from build123d import *

# Parameters (mm, degrees)
EXTRUDE_1_DEPTH     = 50
CHAMFER_1_SIZE      = 5
FILLET_1_R          = 1
SKETCH_2_R          = 12.5
SKETCH_2_R_2        = 2.147801841
CUT_EXTRUDE_1_DEPTH = 84.432542833
CUT_EXTRUDE_2_DEPTH = 80.287617379


with BuildPart() as part:
    # 스케치1 → 보스-돌출1 (new body)
    with BuildSketch(Plane(origin=(0, 0, 0), x_dir=(0, 0, -1), z_dir=(1, 0, 0))):
        with BuildLine():
            Line((-18.568527919, -10.355329949), (31.431472081, -10.355329949))
            ThreePointArc((31.431472081, -10.355329949), (33.552792425, -9.476650293), (34.431472081, -7.355329949))
            Line((34.431472081, -7.355329949), (34.431472081, 40.644670051))
            Line((34.431472081, 40.644670051), (31.431472081, 40.644670051))
            Line((31.431472081, 40.644670051), (31.431472081, -7.355329949))
            Line((31.431472081, -7.355329949), (-18.568527919, -7.355329949))
            Line((-18.568527919, -7.355329949), (-18.568527919, -10.355329949))
        make_face()
    extrude(amount=EXTRUDE_1_DEPTH)

    # 모따기1
    chamfer_1_edges = [part.edges().sort_by_distance(p)[0] for p in [
        (0, -8.855329949, 18.568527919),
        (50, 40.644670051, -32.931472081),
        (50, -8.855329949, 18.568527919),
        (0, 40.644670051, -32.931472081),
    ]]
    chamfer(chamfer_1_edges, length=CHAMFER_1_SIZE)

    # 필렛1
    fillet_1_edges = [part.edges().sort_by_distance(p)[0] for p in [
        (25, -7.355329949, -31.431472081),
    ]]
    fillet(fillet_1_edges, radius=FILLET_1_R)

    # 스케치2 → 컷-돌출1 (cut, through all)
    with BuildSketch(Plane(origin=(0, 0, -34.431472081), x_dir=(-1, 0, 0), z_dir=(0, 0, -1))):
        with Locations((-25, 19.644670051)):
            Circle(SKETCH_2_R)
        with Locations((-37.374368671, 32.019038722)):
            Circle(SKETCH_2_R_2)
        with Locations(Location((-12.625631329, 32.019038722, 0), (0, 0, 90))):
            Circle(SKETCH_2_R_2)
        with Locations((-12.625631329, 7.27030138)):
            Circle(SKETCH_2_R_2)
        with Locations(Location((-37.374368671, 7.27030138, 0), (0, 0, 90))):
            Circle(SKETCH_2_R_2)
    extrude(amount=-CUT_EXTRUDE_1_DEPTH, mode=Mode.SUBTRACT)

    # 스케치3 → 컷-돌출2 (cut, through all)
    with BuildSketch(Plane.XZ.offset(10.355329949)):
        with BuildLine():
            Line((12, 7.568527919), (12, -22.431472081))
            ThreePointArc((12, -22.431472081), (10, -24.431472081), (8, -22.431472081))
            Line((8, -22.431472081), (8, 7.568527919))
            ThreePointArc((8, 7.568527919), (10, 9.568527919), (12, 7.568527919))
        make_face()
        with BuildLine():
            Line((42, 7.568527919), (42, -22.431472081))
            ThreePointArc((42, -22.431472081), (40, -24.431472081), (38, -22.431472081))
            Line((38, -22.431472081), (38, 7.568527919))
            ThreePointArc((38, 7.568527919), (40, 9.568527919), (42, 7.568527919))
        make_face()
    extrude(amount=-CUT_EXTRUDE_2_DEPTH, mode=Mode.SUBTRACT)


solid = part.part
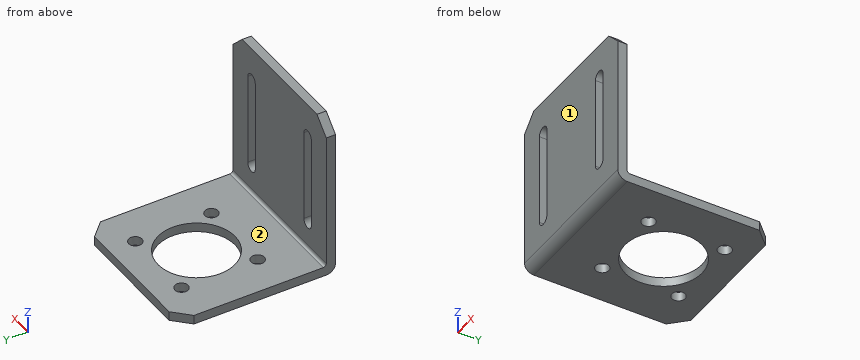
Geometry: final body of the model. Coordinates: model frame, mm. Face numbers are marked on the shaded views. A direction names the side the tool comes from. Round coordinates to 2 decimals unless told otherwise and drop trailing zeros. Order: outer loops, then holes, each group sorted by start corner. A loop starts at its lowest first (then second) coordinate and runs counter-clockwise, first axis right, second up. Notation, with made-up numbers: (85.5, 6) -> (94.5, 6) arc R28 cw to (94.5, 39) -> close; hole circle Ø7 at (28.25, 27.25). An arc over 180 degrees is marked (long way). Put each result on its own line as item: value. Start each with the question number.
Q1. Section C-C on y = 11. Return the cut outline in (x, z), and give its area (3 significant figures).
Q2. Section D-D on x = 16.5. Return the cut outline in (y, z).
Q3. Section B-B on x = 25. Return the cut outline in (y, z), and give its area (3 significant figures).
Q4. Reachability of the marked faces 1 and 2 from +Z, -Z, +X, -X, +Y, -Y: full face, straight path, thin tool, end or side. Return the list, or none.
Q5. First-contact query: pin 1 (6 mm diameter, centred on x = 26, y = 1.5, fed in from +Z); pin 2 (14.5 mm diameter, centred on x = 26, z = 5.5, fed in from +Y). Flat tips, straight axial feed; report the tip coordinate or a pass-through.
Q6. Line query: probe 1 along Y at (x, z) = (26, 13); probe 2 along Z at (x, y) = (47, 37.5); probe 3 along Y at (x, z) = (25, -33.2). Output: solid intervals per line, ascending.
Q7. Section A-A on z = 2.5. Return the cut outline in (x, y), and give its area (3 significant figures).
Ans:
1. outline: (0, -34.43) -> (15.97, -34.43) -> (15.97, -31.43) -> (0, -31.43) -> close; (34.03, -34.43) -> (50, -34.43) -> (50, -31.43) -> (34.03, -31.43) -> close
1. area: 95.8 mm2
2. outline: (-10.36, -31.43) arc R3 ccw to (-7.36, -34.43) -> (10.48, -34.43) -> (10.48, -31.43) -> (-6.36, -31.43) arc R1 cw to (-7.36, -30.43) -> (-7.36, 18.57) -> (-10.36, 18.57) -> close; (28.81, -34.43) -> (40.64, -34.43) -> (40.64, -31.43) -> (28.81, -31.43) -> close
3. outline: (-10.36, -31.43) arc R3 ccw to (-7.36, -34.43) -> (7.14, -34.43) -> (7.14, -31.43) -> (-6.36, -31.43) arc R1 cw to (-7.36, -30.43) -> (-7.36, 18.57) -> (-10.36, 18.57) -> close; (32.14, -34.43) -> (40.64, -34.43) -> (40.64, -31.43) -> (32.14, -31.43) -> close
3. area: 226 mm2
4. face 1: +Z, -Z, +X, -X, -Y
4. face 2: +Z, +X, -X, +Y
5. pin 1: stops at z = -31.43
5. pin 2: stops at y = -7.36
6. probe 1: y = -10.36 to -7.36
6. probe 2: z = -34.43 to -31.43
6. probe 3: y = -9.78 to 7.14, 32.14 to 40.64
7. outline: (0, -10.36) -> (8, -10.36) -> (8, -7.36) -> (0, -7.36) -> close; (12, -10.36) -> (38, -10.36) -> (38, -7.36) -> (12, -7.36) -> close; (42, -10.36) -> (50, -10.36) -> (50, -7.36) -> (42, -7.36) -> close
7. area: 126 mm2
